Source: CAD feature listing. Evaluate the final solid. Frame: model axes, mm. Face numbers are marked on the shaded views. Round coordinates to 2 decimals unless told otherwise and drop trailing zeros. Order: outer loops, then holes, each group sorted by start corner. A loop starts at its lowest first (then second) coordinate and runs counter-clockwise, first axis right, second up. Notation, with made-up numbers: M -12.5,-8 L 23.5,-8 A15 ccw 23.5,-3 Z; hole C -24.75,8 d7. An arc over 180 degrees is marked long. Answer as CSV lines item,"result". Start each with the question number.
Item 1: Section query B-B on z = 0. Return the cut outline in (x, y), plus the area to 3 significant figures.
Item 2: Section query C-C on y = 5.25. Return the cut outline in (x, z), plus the area to 3 significant figures.
Item 3: Line query: line 1 (Z direction, x = 0, y = 2.25); line 2 (Z direction, x = -2, y = 2.5). Output: solid intervals per line, ascending. Write a range as [from, to].
Item 4: Pull-direction query (X, two-part tool) for the marked faces 1, 2, 3 and 4; classes: +X half, -X half, draft (parallel to the pull), parting line (faces both ways), or undercut.
Item 5: Section query A-A on x = 0. Return the cut outline in (y, z).
from build123d import *

# Parameters (mm, degrees)
SKETCH1_W               = 2.5
SKETCH1_H               = 2.5
BOSS_EXTRUDE1_DEPTH     = 2
CUT_EXTRUDE1_DEPTH      = 3.669269563
CUT_EXTRUDE1_DEPTH_BACK = 3.669269563
SKETCH2_R               = 0.5
SCALE1_SCALE            = 6


with BuildPart() as part:
    # Sketch1 → Boss-Extrude1 (new body)
    with BuildSketch(Plane(origin=(0, 0, 0), x_dir=(1, 0, 0), z_dir=(0, 1, 0))):
        Rectangle(SKETCH1_W, SKETCH1_H)
    extrude(amount=BOSS_EXTRUDE1_DEPTH)

    # Sketch2 → Cut-Extrude1 (cut, two sides: drawn at the far end of the back side and taken through both)
    with BuildSketch(Plane(origin=(0, 2, 0), x_dir=(1, 0, 0), z_dir=(0, 1, 0)).offset(-CUT_EXTRUDE1_DEPTH_BACK)):
        with Locations(Location((0, 0, 0), (0, 0, 270))):
            Circle(SKETCH2_R)
    extrude(amount=CUT_EXTRUDE1_DEPTH + CUT_EXTRUDE1_DEPTH_BACK, mode=Mode.SUBTRACT)


with BuildPart() as part_1:
    # Scale1: scaled about (0, 1, 0)
    add(part.part.scale(SCALE1_SCALE).moved(Location((0, -5, 0))))


solid = part_1.part
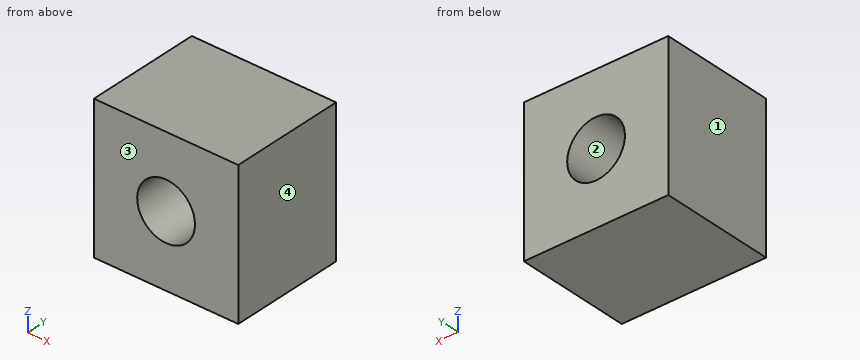
Results:
1,outline,"M -7.5,-5 L -3,-5 L -3,7 L -7.5,7 Z; M 3,-5 L 7.5,-5 L 7.5,7 L 3,7 Z"
1,area,"108 mm^2"
2,outline,"M -7.5,-7.5 L 7.5,-7.5 L 7.5,7.5 L -7.5,7.5 Z; hole C 0,0 d6"
2,area,"197 mm^2"
3,line 1,"[-7.5, -3], [3, 7.5]"
3,line 2,"[-7.5, -2.24], [2.24, 7.5]"
4,face 1,"-X half"
4,face 2,"undercut"
4,face 3,"draft"
4,face 4,"+X half"
5,outline,"M -5,-7.5 L 7,-7.5 L 7,-3 L -5,-3 Z; M -5,3 L 7,3 L 7,7.5 L -5,7.5 Z"
